The listing builds one solid part. Answer for the finished solid, in the listing's coordinates (mm). Face numbers are marked on the shaded views. A direction names the side the tool comes from. Coordinates: 2 decimals unless noted, no trailing zeros. Write each loop counter-clockwise with the first axis right and the second up, starting at its lowest first coordinate (ties: lowest second). Pieces come first, ordered by that corner, then holes. Notation, with made-up numbers: M 37.25,65.5 L 50.25,65.5 A32 ccw 50.25,93.5 Z; hole C 89.5,-23.5 d4. An arc over 180 degrees is marked long. Answer as CSV lines item,"result".
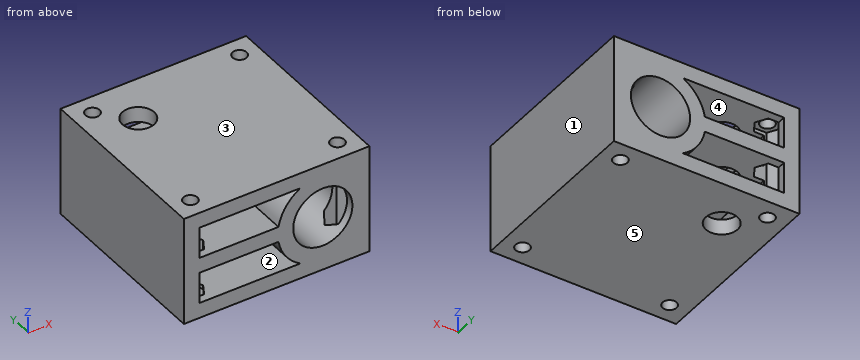
```python
from build123d import *

# Parameters (mm, degrees)
F3_W          = 48.25
F3_H          = 28.25
F3_R          = 7.7
F4_DEPTH      = 24.2
F5_R          = 1.825
F6_DEPTH      = 28.25
F5_R_2        = 4.125
F7_DEPTH      = 28.25
F9_DEPTH      = 13.125
F9_DEPTH_BACK = 9.125


# Not quite as in the source:
# - a feature names something its author has since deleted; it is built from what else it names


with BuildPart() as f4:
    # F3 (on Front) → F4 (new body, symmetric)
    with BuildSketch(Plane.XZ):
        Rectangle(F3_W, F3_H)
        with BuildLine():
            ThreePointArc((23.5277925033, 2), (23.6568686252, 1.0037000824), (23.7, 0))
            ThreePointArc((23.7, 0), (23.6568686252, -1.0037000824), (23.5277925033, -2))
            ThreePointArc((23.5277925033, -2), (22.3372126342, -5.4801491728), (20.125, -8.4186920005))
            Line((20.125, -8.4186920005), (20.125, -10.125))
            Line((20.125, -10.125), (17.8629663994, -10.125))
            ThreePointArc((17.8629663994, -10.125), (15.9935594213, -10.9973398215), (14, -11.5277925033))
            ThreePointArc((14, -11.5277925033), (12, -11.7), (10, -11.5277925033))
            ThreePointArc((10, -11.5277925033), (8.0064405787, -10.9973398215), (6.1370336006, -10.125))
            Line((6.1370336006, -10.125), (-20.125, -10.125))
            Line((-20.125, -10.125), (-20.125, -2))
            Line((-20.125, -2), (-20.125, 2))
            Line((-20.125, 2), (-20.125, 10.125))
            Line((-20.125, 10.125), (6.1370336006, 10.125))
            ThreePointArc((6.1370336006, 10.125), (8.0064405787, 10.9973398215), (10, 11.5277925033))
            ThreePointArc((10, 11.5277925033), (12, 11.7), (14, 11.5277925033))
            ThreePointArc((14, 11.5277925033), (15.9935594213, 10.9973398215), (17.8629663994, 10.125))
            Line((17.8629663994, 10.125), (20.125, 10.125))
            Line((20.125, 10.125), (20.125, 8.4186920005))
            ThreePointArc((20.125, 8.4186920005), (22.3372126342, 5.4801491728), (23.5277925033, 2))
        make_face(mode=Mode.SUBTRACT)
        with BuildLine():
            Line((14, 10.125), (14, 11.5277925033))
            ThreePointArc((14, 11.5277925033), (12, 11.7), (10, 11.5277925033))
            Line((10, 11.5277925033), (10, 10.125))
            Line((10, 10.125), (14, 10.125))
        make_face()
        with BuildLine():
            Line((20.125, 2), (20.125, 8.4186920005))
            ThreePointArc((20.125, 8.4186920005), (19.045826619, 9.3405742466), (17.8629663994, 10.125))
            Line((17.8629663994, 10.125), (14, 10.125))
            Line((14, 10.125), (10, 10.125))
            Line((10, 10.125), (6.1370336006, 10.125))
            ThreePointArc((6.1370336006, 10.125), (2.4024206149, 6.6915222444), (0.4722074967, 2))
            ThreePointArc((0.4722074967, 2), (0.3, 0), (0.4722074967, -2))
            ThreePointArc((0.4722074967, -2), (2.4024206149, -6.6915222444), (6.1370336006, -10.125))
            Line((6.1370336006, -10.125), (10, -10.125))
            Line((10, -10.125), (14, -10.125))
            Line((14, -10.125), (17.8629663994, -10.125))
            ThreePointArc((17.8629663994, -10.125), (19.045826619, -9.3405742466), (20.125, -8.4186920005))
            Line((20.125, -8.4186920005), (20.125, -2))
            Line((20.125, -2), (20.125, 2))
        make_face()
        with Locations((12, 0)):
            Circle(F3_R, mode=Mode.SUBTRACT)
        with BuildLine():
            ThreePointArc((10, -11.5277925033), (12, -11.7), (14, -11.5277925033))
            Line((14, -11.5277925033), (14, -10.125))
            Line((14, -10.125), (10, -10.125))
            Line((10, -10.125), (10, -11.5277925033))
        make_face()
        with BuildLine():
            ThreePointArc((0.4722074967, -2), (0.3, 0), (0.4722074967, 2))
            Line((0.4722074967, 2), (-20.125, 2))
            Line((-20.125, 2), (-20.125, -2))
            Line((-20.125, -2), (0.4722074967, -2))
        make_face()
        with BuildLine():
            ThreePointArc((23.5277925033, -2), (23.6568686252, -1.0037000824), (23.7, 0))
            ThreePointArc((23.7, 0), (23.6568686252, 1.0037000824), (23.5277925033, 2))
            Line((23.5277925033, 2), (20.125, 2))
            Line((20.125, 2), (20.125, -2))
            Line((20.125, -2), (23.5277925033, -2))
        make_face()
        with BuildLine():
            Line((20.125, 2), (23.5277925033, 2))
            ThreePointArc((23.5277925033, 2), (22.3372126342, 5.4801491728), (20.125, 8.4186920005))
            Line((20.125, 8.4186920005), (20.125, 2))
        make_face()
        with BuildLine():
            ThreePointArc((20.125, -8.4186920005), (22.3372126342, -5.4801491728), (23.5277925033, -2))
            Line((23.5277925033, -2), (20.125, -2))
            Line((20.125, -2), (20.125, -8.4186920005))
        make_face()
        with BuildLine():
            Line((14, 10.125), (17.8629663994, 10.125))
            ThreePointArc((17.8629663994, 10.125), (15.9935594213, 10.9973398215), (14, 11.5277925033))
            Line((14, 11.5277925033), (14, 10.125))
        make_face()
        with BuildLine():
            Line((10, 10.125), (10, 11.5277925033))
            ThreePointArc((10, 11.5277925033), (8.0064405787, 10.9973398215), (6.1370336006, 10.125))
            Line((6.1370336006, 10.125), (10, 10.125))
        make_face()
        with BuildLine():
            ThreePointArc((17.8629663994, 10.125), (19.045826619, 9.3405742466), (20.125, 8.4186920005))
            Line((20.125, 8.4186920005), (20.125, 10.125))
            Line((20.125, 10.125), (17.8629663994, 10.125))
        make_face()
        with BuildLine():
            Line((20.125, -10.125), (20.125, -8.4186920005))
            ThreePointArc((20.125, -8.4186920005), (19.045826619, -9.3405742466), (17.8629663994, -10.125))
            Line((17.8629663994, -10.125), (20.125, -10.125))
        make_face()
        with BuildLine():
            ThreePointArc((14, -11.5277925033), (15.9935594213, -10.9973398215), (17.8629663994, -10.125))
            Line((17.8629663994, -10.125), (14, -10.125))
            Line((14, -10.125), (14, -11.5277925033))
        make_face()
        with BuildLine():
            ThreePointArc((6.1370336006, -10.125), (8.0064405787, -10.9973398215), (10, -11.5277925033))
            Line((10, -11.5277925033), (10, -10.125))
            Line((10, -10.125), (6.1370336006, -10.125))
        make_face()
    extrude(amount=F4_DEPTH, both=True)

    # F5 (on face) → F6 (cut)
    with BuildSketch(Plane(origin=(0, 0, -14.125), x_dir=(1, 0, 0), z_dir=(0, 0, -1))):
        with Locations((-19.125, 19.2)):
            Circle(F5_R)
        with Locations((19.125, 19.2)):
            Circle(F5_R)
        with Locations((19.125, -19.2)):
            Circle(F5_R)
        with Locations((-19.125, -19.2)):
            Circle(F5_R)
    extrude(amount=-F6_DEPTH, mode=Mode.SUBTRACT)

    # F5 (on face) → F7 (cut)
    with BuildSketch(Plane(origin=(0, 0, -14.125), x_dir=(1, 0, 0), z_dir=(0, 0, -1))):
        with Locations((-12, -12)):
            Circle(F5_R_2)
    extrude(amount=-F7_DEPTH, mode=Mode.SUBTRACT)

    # F8 (on face) → F9 (cut, two sides)
    with BuildSketch(Plane.XY.offset(2)) as f9_sk:
        Polygon((20.7848820239, -16.325), (17.4651179761, -16.325), (15.8052359522, -19.2), (17.4651179761, -22.075), (20.7848820239, -22.075), (22.4447640478, -19.2), align=None)
        Polygon((17.4651179761, 16.325), (20.7848820239, 16.325), (22.4447640478, 19.2), (20.7848820239, 22.075), (17.4651179761, 22.075), (15.8052359522, 19.2), align=None)
        Polygon((-20.7848820239, 16.325), (-17.4651179761, 16.325), (-15.8052359522, 19.2), (-17.4651179761, 22.075), (-20.7848820239, 22.075), (-22.4447640478, 19.2), align=None)
        Polygon((-17.4651179761, -16.325), (-20.7848820239, -16.325), (-22.4447640478, -19.2), (-20.7848820239, -22.075), (-17.4651179761, -22.075), (-15.8052359522, -19.2), align=None)
    extrude(amount=-F9_DEPTH, mode=Mode.SUBTRACT)
    extrude(f9_sk.sketch, amount=F9_DEPTH_BACK, mode=Mode.SUBTRACT)


solid = f4.part
```
Q1. Find section C-C (x = -12). Give the vertices of the cut face in (y, z) (3 decimals).
Output:
outline,"M -24.2,-14.125 L 7.875,-14.125 L 7.875,-10.125 L -24.2,-10.125 Z; M -24.2,-2 L 7.875,-2 L 7.875,2 L -24.2,2 Z; M -24.2,10.125 L 7.875,10.125 L 7.875,14.125 L -24.2,14.125 Z; M 16.125,-14.125 L 24.2,-14.125 L 24.2,-10.125 L 16.125,-10.125 Z; M 16.125,-2 L 24.2,-2 L 24.2,2 L 16.125,2 Z; M 16.125,10.125 L 24.2,10.125 L 24.2,14.125 L 16.125,14.125 Z"
Q2. A flat-ended cylindrical pin translates along its axis: pin 1 Ø2 at (x, y) = (-19.125, -19.2) entering from -Z. Find the tip coordinate at first contact, or state that the pin passes through.
Output:
pin 1,"through"
Q3. Find section A-A (z = 0). Count the separate pieces of the cut face and the enclosed holes in it, and give its area (3 significant figures).
Output:
separate pieces,"2"
enclosed holes,"3"
area,"1,460 mm2"
Q4. For the marked faces 4 and 5, determine the directions among +Z, -Z, +X, -X, +Y, -Y from which every point of the face is accessible in a straight line to the end or side of a thin tool.
Output:
face 4,"+Y, -Y"
face 5,"-Z, +X, -X, +Y, -Y"
Q5. Find section D-D (y = 9). Give the vertices of the cut face in (x, z) (3 decimals).
Output:
outline,"M -24.125,-14.125 L -14.831,-14.125 L -14.831,-10.125 L -20.125,-10.125 L -20.125,-2 L -14.831,-2 L -14.831,2 L -20.125,2 L -20.125,10.125 L -14.831,10.125 L -14.831,14.125 L -24.125,14.125 Z; M -9.169,-14.125 L 24.125,-14.125 L 24.125,14.125 L -9.169,14.125 L -9.169,10.125 L 6.137,10.125 A11.7 ccw 0.472,2 L -9.169,2 L -9.169,-2 L 0.472,-2 A11.7 ccw 6.137,-10.125 L -9.169,-10.125 Z; hole C 12,0 d15.4"
Q6. Straight lines are drawn through the part: line 1 (Y direction, x = -18.5, z = 1.5) (3 decimals); line 2 (X direction, y = -19.2, z = -13.45) (3 decimals); line 3 (Z direction, x = -20, y = -15) (3 decimals). For each, find the intervals that lie inside material, in ascending order.
Output:
line 1,"-24.2 to -22.075, -16.325 to 16.325, 22.075 to 24.2"
line 2,"-24.125 to -20.95, -17.3 to 17.3, 20.95 to 24.125"
line 3,"-14.125 to -10.125, -2 to 2, 10.125 to 14.125"
Q7. Find section B-B (x = -6.5). Give the vertices of the cut face in (y, z) (3 decimals).
Output:
outline,"M -24.2,-14.125 L 24.2,-14.125 L 24.2,-10.125 L -24.2,-10.125 Z; M -24.2,-2 L 24.2,-2 L 24.2,2 L -24.2,2 Z; M -24.2,10.125 L 24.2,10.125 L 24.2,14.125 L -24.2,14.125 Z"
Q8. The mould has two halves that part along Z. Classify the marked faces 1, 2 and 3: pulls with the +Z half, pulls with the -Z half, needs draft (parallel to the pull), parting line crosses it, or undercut.
Output:
face 1,"needs draft"
face 2,"undercut"
face 3,"pulls with the +Z half"
